Geometry check sheet. Reference: the model listing, model coordinates, mm. Face numbers are marked on the shaded views. A direction names the side the tool comes from. Coordinates: 2 decimals unless noted, no trailing zeros. Write each loop counter-clockwise with the first axis right and the second up, starting at its lowest first coordinate (ties: lowest second). Pieces come first, ordered by that corner, then holes. Notation, with made-up numbers: (22.5, -12.75) -> (33.5, -12.75) arc R25 cw to (33.5, 13.25) -> close; hole circle Ø6 at (-20.5, 70). An arc over 180 degrees is marked (long way). Use a Markdown table: item, result.
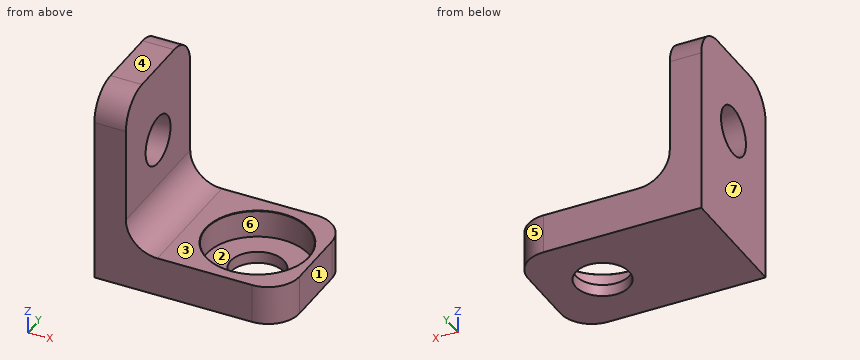
```python
from build123d import *

# Parameters (mm, degrees)
ESBO_O1_W                = 12
ESBO_O1_H                = 8
RESSALTO_EXTRUS_O1_DEPTH = 2.5
ESBO_O3_W                = 2
ESBO_O3_H                = 8
RESSALTO_EXTRUS_O2_DEPTH = 10
FILETE1_R                = 2
FILETE2_R                = 2
CORTE_EXTRUS_O2_REACH    = 19.095
ESBO_O6_R                = 1.55


with BuildPart() as part:
    # Esboço1 → Ressalto-extrusão1 (new body)
    with BuildSketch(Plane.XY):
        with Locations((-6, 2)):
            Rectangle(ESBO_O1_W, ESBO_O1_H)
    extrude(amount=RESSALTO_EXTRUS_O1_DEPTH)

    # Esboço3 → Ressalto-extrusão2 (add)
    with BuildSketch(Plane.XY.offset(2.5)):
        with Locations((-11, 2)):
            Rectangle(ESBO_O3_W, ESBO_O3_H)
    extrude(amount=RESSALTO_EXTRUS_O2_DEPTH)

    # Esboço10 → Rebaixo para parafuso com cabeça redonda de M33 (revolve, cut)
    with BuildSketch(Plane(origin=(-3.7, 2, 2.5), x_dir=(0, -1, 0), z_dir=(1, 0, 0))):
        Polygon((0, 0), (0, 2.5), (1.7, 2.5), (1.7, 1.75), (3.25, 1.75), (3.25, 0.025), (3.275, 0), align=None)
    revolve(axis=Axis((-3.7, 2, 8.85), (0, 0, -1)), mode=Mode.SUBTRACT)

    # Filete1
    filete1_edges = [part.edges().sort_by_distance(p)[0] for p in [
        (-10, 2, 2.5),
    ]]
    fillet(filete1_edges, radius=FILETE1_R)

    # Filete2
    filete2_edges = [part.edges().sort_by_distance(p)[0] for p in [
        (-11, -2, 12.5),
        (-11, 6, 12.5),
        (0, 6, 1.25),
        (0, -2, 1.25),
    ]]
    fillet(filete2_edges, radius=FILETE2_R)

    # Esboço6 → Corte-extrusão2 (cut, up to next)
    with BuildSketch(Plane(origin=(-10, 0, 0), x_dir=(0, 0, -1), z_dir=(1, 0, 0)), mode=Mode.PRIVATE) as corte_extrus_o2_sk1:
        with Locations(Location((-7.55, 2, 0), (0, 0, 90))):
            Circle(ESBO_O6_R)
    corte_extrus_o2_tool1 = extrude(corte_extrus_o2_sk1.sketch, amount=-CORTE_EXTRUS_O2_REACH, mode=Mode.PRIVATE) & part.part
    add(corte_extrus_o2_tool1.solids().sort_by_distance((-10, 2, 7.55))[0], mode=Mode.SUBTRACT)


solid = part.part
```
Item 1: Thickness scan on L1, parallel to Y at x = -11, z = 7.5; L2, parallel to Z at x = -11.1, y = 2; L3, parallel to Z at x = -1, y = 0.5. Record the ranges inside material, lowest first. Write a range as [from, to].
Answer block:
| item | result |
|---|---|
| L1 | y = [-2, 0.45], [3.55, 6] |
| L2 | z = [0, 6], [9.1, 12.5] |
| L3 | z = [0, 0.75] |
Item 2: Section check B-B on x = -3.7. Record the boundary of the cut face in (y, z) (3 decimals).
Answer block:
| item | result |
|---|---|
| outline | (-2, 0) -> (0.3, 0) -> (0.3, 0.75) -> (-1.25, 0.75) -> (-1.25, 2.475) -> (-1.275, 2.5) -> (-2, 2.5) -> close; (3.7, 0) -> (6, 0) -> (6, 2.5) -> (5.275, 2.5) -> (5.25, 2.475) -> (5.25, 0.75) -> (3.7, 0.75) -> close |
Item 3: Section check A-A on z = 7.55. Record the boundary of the cut face in (x, y).
Answer block:
| item | result |
|---|---|
| outline | (-12, -2) -> (-10, -2) -> (-10, 0.45) -> (-12, 0.45) -> close; (-12, 3.55) -> (-10, 3.55) -> (-10, 6) -> (-12, 6) -> close |
Item 4: Section check D-D on x = -10.25. Record the boundary of the cut face in (y, z).
Answer block:
| item | result |
|---|---|
| outline | (-2, 0) -> (6, 0) -> (6, 10.5) arc R2 ccw to (4, 12.5) -> (0, 12.5) arc R2 ccw to (-2, 10.5) -> close; hole circle Ø3.1 at (2, 7.55) |
Item 5: Depth check by flat-ended pin: P1, Ø2.5, axis at y = 1, z = 6.5, coming from the +X side; P2, Ø3, axis at x = -7, y = 4.5, coming from the +Z side; P3, Ø2, axis at x = -4.5, y = 3.5, coming from the +Z side. Enter the tip coordinate at first touch or a pass-through.
Answer block:
| item | result |
|---|---|
| P1 | stops at x = -10 |
| P2 | stops at z = 2.56 |
| P3 | stops at z = 0.75 |
Item 6: Section check C-C on y = 2. Record the boundary of the cut face in (x, z) (3 decimals).
Answer block:
| item | result |
|---|---|
| outline | (-12, 0) -> (-5.4, 0) -> (-5.4, 0.75) -> (-6.95, 0.75) -> (-6.95, 2.475) -> (-6.975, 2.5) -> (-8, 2.5) arc R2 cw to (-10, 4.5) -> (-10, 6) -> (-12, 6) -> close; (-12, 9.1) -> (-10, 9.1) -> (-10, 12.5) -> (-12, 12.5) -> close; (-2, 0) -> (0, 0) -> (0, 2.5) -> (-0.425, 2.5) -> (-0.45, 2.475) -> (-0.45, 0.75) -> (-2, 0.75) -> close |
Item 7: Tool access check on the marked faces 1, 2 and 3. Record the directions out of +Z, -Z, +X, -X, +Y, -Y that give a thin tool (end or side, any length) a straight path to the whole face; none if there is none.
Answer block:
| item | result |
|---|---|
| face 1 | +Z, -Z, +X, +Y, -Y |
| face 2 | +Z |
| face 3 | +Z, +X, +Y, -Y |
Item 8: Mould release check, pull along X, two halves, no side actions. Record for the marked faces 4, 5, 6 and 7: +X half, -X half, draft (parallel to the pull), parting line (faces both ways), or undercut.
Answer block:
| item | result |
|---|---|
| face 4 | draft |
| face 5 | +X half |
| face 6 | undercut |
| face 7 | -X half |
